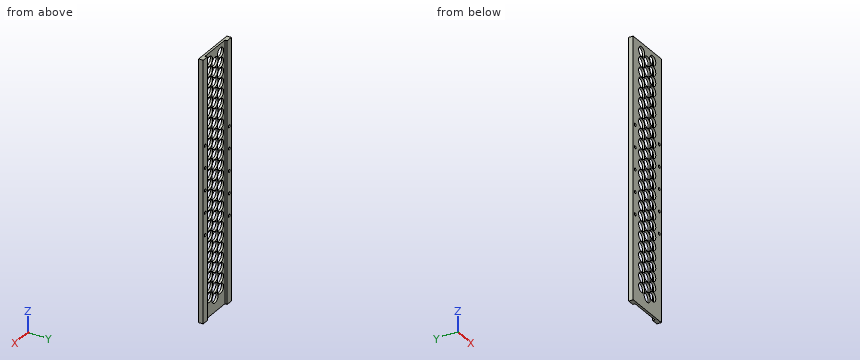
from build123d import *

# Parameters (mm, degrees)
CELL_BLOCK_SKETCH_W = 71.300566034
CELL_BLOCK_SKETCH_H = 589.575
BOSS_EXTRUDE1_DEPTH = 5
SKETCH1_R           = 10.875
CUT_EXTRUDE2_DEPTH  = 5
SKETCH3_W           = 15
SKETCH3_H           = 589.575
BOSS_EXTRUDE3_DEPTH = 10
SKETCH4_R           = 3.25
CUT_EXTRUDE3_DEPTH  = 10


with BuildPart() as part:
    # Cell Block Sketch → Boss-Extrude1 (new body)
    with BuildSketch(Plane(origin=(0, 0, 0), x_dir=(1, 0, 0), z_dir=(0, 1, 0))):
        Rectangle(CELL_BLOCK_SKETCH_W, CELL_BLOCK_SKETCH_H)
    extrude(amount=BOSS_EXTRUDE1_DEPTH)

    # Sketch1 → Cut-Extrude2 (cut)
    with BuildSketch(Plane(origin=(0, 5, 0), x_dir=(1, 0, 0), z_dir=(0, 1, 0))):
        with Locations(Location((-19.875283017, 252.5375, 0), (0, 0, 270))):
            Circle(SKETCH1_R)
        with Locations(Location((0, 264.0125, 0), (0, 0, 270))):
            Circle(SKETCH1_R)
        with Locations(Location((19.875283017, 252.5375, 0), (0, 0, 270))):
            Circle(SKETCH1_R)
        with Locations(Location((-19.875283017, 229.5875, 0), (0, 0, 270))):
            Circle(SKETCH1_R)
        with Locations(Location((0, 241.0625, 0), (0, 0, 270))):
            Circle(SKETCH1_R)
        with Locations(Location((19.875283017, 229.5875, 0), (0, 0, 270))):
            Circle(SKETCH1_R)
        with Locations(Location((-19.875283017, 206.6375, 0), (0, 0, 270))):
            Circle(SKETCH1_R)
        with Locations(Location((0, 218.1125, 0), (0, 0, 270))):
            Circle(SKETCH1_R)
        with Locations(Location((19.875283017, 206.6375, 0), (0, 0, 270))):
            Circle(SKETCH1_R)
        with Locations(Location((-19.875283017, 183.6875, 0), (0, 0, 270))):
            Circle(SKETCH1_R)
        with Locations(Location((0, 195.1625, 0), (0, 0, 270))):
            Circle(SKETCH1_R)
        with Locations(Location((19.875283017, 183.6875, 0), (0, 0, 270))):
            Circle(SKETCH1_R)
        with Locations(Location((-19.875283017, 160.7375, 0), (0, 0, 270))):
            Circle(SKETCH1_R)
        with Locations(Location((0, 172.2125, 0), (0, 0, 270))):
            Circle(SKETCH1_R)
        with Locations(Location((19.875283017, 160.7375, 0), (0, 0, 270))):
            Circle(SKETCH1_R)
        with Locations(Location((-19.875283017, 137.7875, 0), (0, 0, 270))):
            Circle(SKETCH1_R)
        with Locations(Location((0, 149.2625, 0), (0, 0, 270))):
            Circle(SKETCH1_R)
        with Locations(Location((19.875283017, 137.7875, 0), (0, 0, 270))):
            Circle(SKETCH1_R)
        with Locations(Location((-19.875283017, 114.8375, 0), (0, 0, 270))):
            Circle(SKETCH1_R)
        with Locations(Location((0, 126.3125, 0), (0, 0, 270))):
            Circle(SKETCH1_R)
        with Locations(Location((19.875283017, 114.8375, 0), (0, 0, 270))):
            Circle(SKETCH1_R)
        with Locations(Location((-19.875283017, 91.8875, 0), (0, 0, 270))):
            Circle(SKETCH1_R)
        with Locations(Location((0, 103.3625, 0), (0, 0, 270))):
            Circle(SKETCH1_R)
        with Locations(Location((19.875283017, 91.8875, 0), (0, 0, 270))):
            Circle(SKETCH1_R)
        with Locations(Location((-19.875283017, 68.9375, 0), (0, 0, 270))):
            Circle(SKETCH1_R)
        with Locations(Location((0, 80.4125, 0), (0, 0, 270))):
            Circle(SKETCH1_R)
        with Locations(Location((19.875283017, 68.9375, 0), (0, 0, 270))):
            Circle(SKETCH1_R)
        with Locations(Location((-19.875283017, 45.9875, 0), (0, 0, 270))):
            Circle(SKETCH1_R)
        with Locations(Location((0, 57.4625, 0), (0, 0, 270))):
            Circle(SKETCH1_R)
        with Locations(Location((19.875283017, 45.9875, 0), (0, 0, 270))):
            Circle(SKETCH1_R)
        with Locations(Location((-19.875283017, 23.0375, 0), (0, 0, 270))):
            Circle(SKETCH1_R)
        with Locations(Location((0, 34.5125, 0), (0, 0, 270))):
            Circle(SKETCH1_R)
        with Locations(Location((19.875283017, 23.0375, 0), (0, 0, 270))):
            Circle(SKETCH1_R)
        with Locations(Location((-19.875283017, 0.0875, 0), (0, 0, 270))):
            Circle(SKETCH1_R)
        with Locations(Location((0, 11.5625, 0), (0, 0, 270))):
            Circle(SKETCH1_R)
        with Locations(Location((19.875283017, 0.0875, 0), (0, 0, 270))):
            Circle(SKETCH1_R)
        with Locations(Location((-19.875283017, -22.8625, 0), (0, 0, 270))):
            Circle(SKETCH1_R)
        with Locations(Location((0, -11.3875, 0), (0, 0, 270))):
            Circle(SKETCH1_R)
        with Locations(Location((19.875283017, -22.8625, 0), (0, 0, 270))):
            Circle(SKETCH1_R)
        with Locations(Location((-19.875283017, -45.8125, 0), (0, 0, 270))):
            Circle(SKETCH1_R)
        with Locations(Location((0, -34.3375, 0), (0, 0, 270))):
            Circle(SKETCH1_R)
        with Locations(Location((19.875283017, -45.8125, 0), (0, 0, 270))):
            Circle(SKETCH1_R)
        with Locations(Location((-19.875283017, -68.7625, 0), (0, 0, 270))):
            Circle(SKETCH1_R)
        with Locations(Location((0, -57.2875, 0), (0, 0, 270))):
            Circle(SKETCH1_R)
        with Locations(Location((19.875283017, -68.7625, 0), (0, 0, 270))):
            Circle(SKETCH1_R)
        with Locations(Location((-19.875283017, -91.7125, 0), (0, 0, 270))):
            Circle(SKETCH1_R)
        with Locations(Location((0, -80.2375, 0), (0, 0, 270))):
            Circle(SKETCH1_R)
        with Locations(Location((19.875283017, -91.7125, 0), (0, 0, 270))):
            Circle(SKETCH1_R)
        with Locations(Location((-19.875283017, -114.6625, 0), (0, 0, 270))):
            Circle(SKETCH1_R)
        with Locations(Location((0, -103.1875, 0), (0, 0, 270))):
            Circle(SKETCH1_R)
        with Locations(Location((19.875283017, -114.6625, 0), (0, 0, 270))):
            Circle(SKETCH1_R)
        with Locations(Location((-19.875283017, -137.6125, 0), (0, 0, 270))):
            Circle(SKETCH1_R)
        with Locations(Location((0, -126.1375, 0), (0, 0, 270))):
            Circle(SKETCH1_R)
        with Locations(Location((19.875283017, -137.6125, 0), (0, 0, 270))):
            Circle(SKETCH1_R)
        with Locations(Location((-19.875283017, -160.5625, 0), (0, 0, 270))):
            Circle(SKETCH1_R)
        with Locations(Location((0, -149.0875, 0), (0, 0, 270))):
            Circle(SKETCH1_R)
        with Locations(Location((19.875283017, -160.5625, 0), (0, 0, 270))):
            Circle(SKETCH1_R)
        with Locations(Location((-19.875283017, -183.5125, 0), (0, 0, 270))):
            Circle(SKETCH1_R)
        with Locations(Location((0, -172.0375, 0), (0, 0, 270))):
            Circle(SKETCH1_R)
        with Locations(Location((19.875283017, -183.5125, 0), (0, 0, 270))):
            Circle(SKETCH1_R)
        with Locations(Location((-19.875283017, -206.4625, 0), (0, 0, 270))):
            Circle(SKETCH1_R)
        with Locations(Location((0, -194.9875, 0), (0, 0, 270))):
            Circle(SKETCH1_R)
        with Locations(Location((19.875283017, -206.4625, 0), (0, 0, 270))):
            Circle(SKETCH1_R)
        with Locations(Location((-19.875283017, -229.4125, 0), (0, 0, 270))):
            Circle(SKETCH1_R)
        with Locations(Location((0, -217.9375, 0), (0, 0, 270))):
            Circle(SKETCH1_R)
        with Locations(Location((19.875283017, -229.4125, 0), (0, 0, 270))):
            Circle(SKETCH1_R)
        with Locations(Location((-19.875283017, -252.3625, 0), (0, 0, 270))):
            Circle(SKETCH1_R)
        with Locations(Location((0, -240.8875, 0), (0, 0, 270))):
            Circle(SKETCH1_R)
        with Locations(Location((19.875283017, -252.3625, 0), (0, 0, 270))):
            Circle(SKETCH1_R)
        with Locations(Location((-19.875283017, -275.3125, 0), (0, 0, 270))):
            Circle(SKETCH1_R)
        with Locations(Location((0, -263.8375, 0), (0, 0, 270))):
            Circle(SKETCH1_R)
        with Locations(Location((19.875283017, -275.3125, 0), (0, 0, 270))):
            Circle(SKETCH1_R)
    extrude(amount=-CUT_EXTRUDE2_DEPTH, mode=Mode.SUBTRACT)

    # Sketch3 → Boss-Extrude3 (add)
    with BuildSketch(Plane(origin=(0, 0, 0), x_dir=(1, 0, 0), z_dir=(0, 1, 0))):
        with Locations((-43.150283017, 0)):
            Rectangle(SKETCH3_W, SKETCH3_H)
    boss_extrude3 = extrude(amount=BOSS_EXTRUDE3_DEPTH)

    # Mirror1: Boss-Extrude3 across plane
    add(boss_extrude3.mirror(Plane(origin=(0, 0, 0), x_dir=(0, 0, 1), z_dir=(1, 0, 0))))

    # Sketch4 → Cut-Extrude3 (cut)
    with BuildSketch(Plane(origin=(0, 10, 0), x_dir=(1, 0, 0), z_dir=(0, 1, 0))):
        with Locations(Location((-43.150283017, 0, 0), (0, 0, 270))):
            Circle(SKETCH4_R)
        with Locations(Location((-43.150283017, -50, 0), (0, 0, 270))):
            Circle(SKETCH4_R)
        with Locations(Location((-43.150283017, -100, 0), (0, 0, 270))):
            Circle(SKETCH4_R)
        with Locations(Location((-43.150283017, 50, 0), (0, 0, 270))):
            Circle(SKETCH4_R)
        with Locations(Location((-43.150283017, 100, 0), (0, 0, 270))):
            Circle(SKETCH4_R)
    cut_extrude3 = extrude(amount=-CUT_EXTRUDE3_DEPTH, mode=Mode.SUBTRACT)

    # Mirror2: Cut-Extrude3 across plane
    add(cut_extrude3.mirror(Plane(origin=(0, 0, 0), x_dir=(0, 0, 1), z_dir=(1, 0, 0))), mode=Mode.SUBTRACT)


solid = part.part
Model file for the job. Use its own axes, mm. Round coordinates to 2 decimals unless told otherwise and drop trailing zeros. Answer as CSV lines item,"result". Start each with the question number.
1) Pin check, flat tips, straight feed: P1, Ø1.5, axis at x = 24, z = 59, coming from the +Y side; P2, Ø13, axis at x = 19.88, z = 137.61, coming from the +Y side. Stop position of each tip, or through.
2) Slice it at A-A (y = 7.25). State how many separate pieces and enclosed holes the cut face has, plus the area to 3 significant figures.
3) Probe line 1 along X through (y, z) = (7.75, 99.5); line 2 along Z through (x, y) = (43, 6.5); line 3 along X through (y, z) = (1.75, 66). List the from-to ranges inside material, lowest first.
Filled in:
1,P1,"stops at y = 5"
1,P2,"passes through"
2,separate pieces,"2"
2,enclosed holes,"10"
2,area,"17,400 mm2"
3,line 1,"x = -50.65 to -46.36, -39.94 to -35.65, 35.65 to 39.94, 46.36 to 50.65"
3,line 2,"z = -294.79 to -103.25, -96.75 to -53.25, -46.75 to -3.25, 3.25 to 46.75, 53.25 to 96.75, 103.25 to 294.79"
3,line 3,"x = -50.65 to -30.39, -9.36 to -6.51, 6.51 to 9.36, 30.39 to 50.65"
